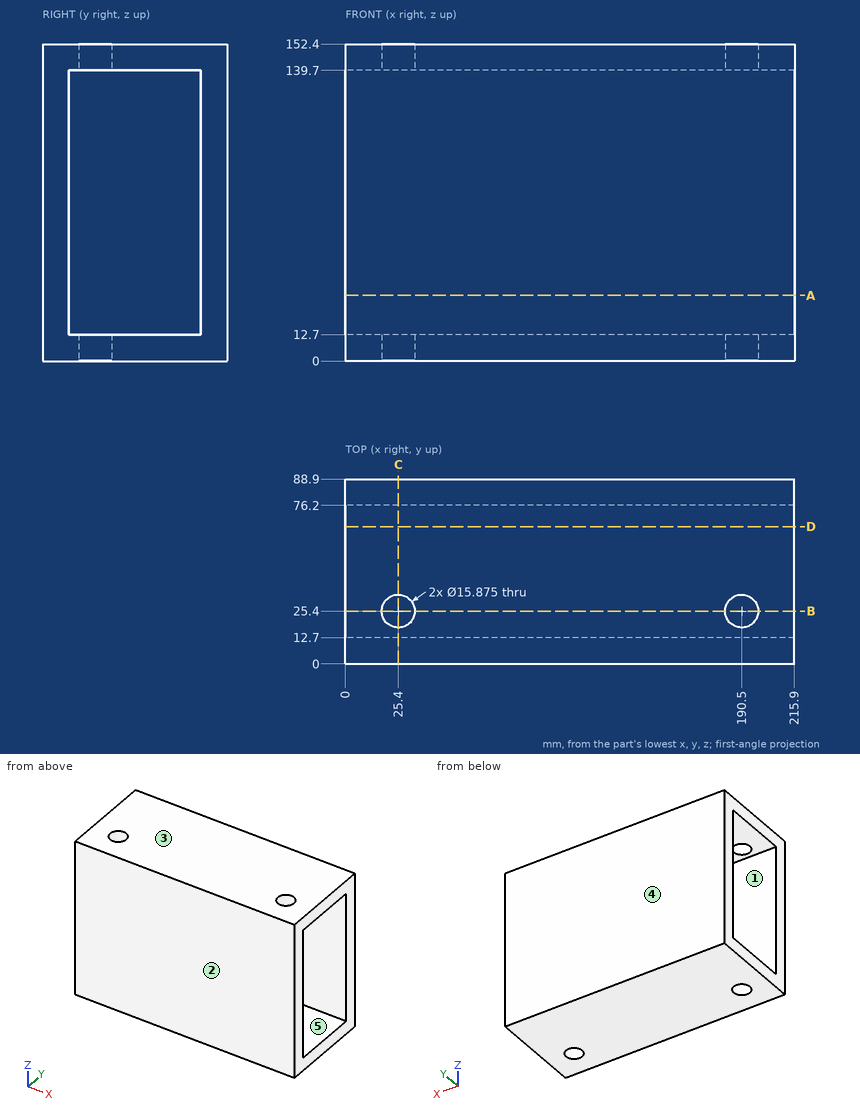
Check sheet for the drawn part. Datum: minimum x, y, z corner. Units: mm. A direction names the side the tool comes from. Give positions to 0.01 mm unless a question says otherwise; leave off trailing zeros. Order: outer loops, then holes, each group sorted by start corner. A loop starts at its lowest first (then second) coordinate and runs counter-clockwise, first axis right, second up. Notation, with made-up numbers: (88.25, 68.25) - (112.25, 68.25) arc R11 ccw to (112.25, 77.25) - close; hole circle Ø8 at (16, 62). An arc over 180 degrees is marked (long way). Answer in a Markdown table with one row per item. Add a question column.
Q1. Gauge pin test, flat ends, axial feed: pin 1 (5 mm diameter, centred on y = 11, z = 18, fed in from -X); pin 2 (14.5 mm diameter, centred on x = 190.5, y = 25.4, fed in from -Z). Record the tip position at first contact, or that the pin passes through.
Q2. Cross-section at D-D, the plane y = 66. Enter the section's corners in (x, z), then the cut area to 3 significant figures.
Q3. Cross-section at B-B, the plane y = 25.4. Enter the section's corners in (x, z).
Q4. Mould release check, pull along Z, two halves, no side actions. Record for the marked faces 3, 4 and 5: pulls with the +Z half, pulls with the -Z half, needs draft (parallel to the pull), parting line crosses it, or undercut.
Q5. Material ranges on probe 1 along X at (y, z) = (25, 146); probe 2 along Z at (x, y) = (184, 64.5); probe 3 along Y at (x, z) = (52.5, 58.5), recorded low to high. Write a range as from..to.
Q6. Tool access check on the marked faces 1 and 2. Record the directions out of +Z, -Z, +X, -X, +Y, -Y that give a thin tool (end or side, any length) a straight path to the whole face; none if there is none.
Q7. Cross-section at C-C, the plane x = 25.4. Enter the section's corners in (y, z), then the cut area to 3 significant figures.
Q8. Cross-section at A-A, the plane z = 31.5. Enter the section's corners in (x, y), then the cut area to 3 significant figures.
Check values:
| question | item | result |
|---|---|---|
| 1 | pin 1 | stops at x = 0 |
| 1 | pin 2 | passes through |
| 2 | outline | (0, 0) - (215.9, 0) - (215.9, 12.7) - (0, 12.7) - close; (0, 139.7) - (215.9, 139.7) - (215.9, 152.4) - (0, 152.4) - close |
| 2 | area | 5,480 mm^2 |
| 3 | outline | (0, 0) - (17.46, 0) - (17.46, 12.7) - (0, 12.7) - close; (0, 139.7) - (17.46, 139.7) - (17.46, 152.4) - (0, 152.4) - close; (33.34, 0) - (182.56, 0) - (182.56, 12.7) - (33.34, 12.7) - close; (33.34, 139.7) - (182.56, 139.7) - (182.56, 152.4) - (33.34, 152.4) - close; (198.44, 0) - (215.9, 0) - (215.9, 12.7) - (198.44, 12.7) - close; (198.44, 139.7) - (215.9, 139.7) - (215.9, 152.4) - (198.44, 152.4) - close |
| 4 | face 3 | pulls with the +Z half |
| 4 | face 4 | needs draft |
| 4 | face 5 | undercut |
| 5 | probe 1 | x = 0..17.47, 33.33..182.57, 198.43..215.9 |
| 5 | probe 2 | z = 0..12.7, 139.7..152.4 |
| 5 | probe 3 | y = 0..12.7, 76.2..88.9 |
| 6 | face 1 | +X, -X |
| 6 | face 2 | +Z, -Z, +X, -X, -Y |
| 7 | outline | (0, 0) - (17.46, 0) - (17.46, 12.7) - (12.7, 12.7) - (12.7, 139.7) - (17.46, 139.7) - (17.46, 152.4) - (0, 152.4) - close; (33.34, 0) - (88.9, 0) - (88.9, 152.4) - (33.34, 152.4) - (33.34, 139.7) - (76.2, 139.7) - (76.2, 12.7) - (33.34, 12.7) - close |
| 7 | area | 5,080 mm^2 |
| 8 | outline | (0, 0) - (215.9, 0) - (215.9, 12.7) - (0, 12.7) - close; (0, 76.2) - (215.9, 76.2) - (215.9, 88.9) - (0, 88.9) - close |
| 8 | area | 5,480 mm^2 |
